from build123d import *

# Parameters (mm, degrees)
CROQUIS1_R              = 10.668
SALIENTE_EXTRUIR1_DEPTH = 5
CROQUIS7_W              = 2
CROQUIS7_H              = 8
CORTAR_EXTRUIR5_DEPTH   = 44.28049503
SALIENTE_EXTRUIR3_DEPTH = 10
CORTAR_EXTRUIR6_REACH   = 53.457
CROQUIS9_R              = 2.25
SALIENTE_EXTRUIR4_DEPTH = 10
CROQUIS11_W             = 29.05
CROQUIS11_H             = 10
SALIENTE_EXTRUIR5_DEPTH = 5
CORTAR_EXTRUIR7_REACH   = 52.054
SALIENTE_EXTRUIR6_DEPTH = 8.51
CORTAR_EXTRUIR8_REACH   = 58.395
SALIENTE_EXTRUIR7_DEPTH = 5


with BuildPart() as part:
    # Croquis1 → Saliente-Extruir1 (new, symmetric)
    with BuildSketch(Plane(origin=(0, 0, 0), x_dir=(1, 0, 0), z_dir=(0, 1, 0))):
        with BuildLine():
            Line((14.525, 0), (-14.525, 0))
            Line((-14.525, 0), (-14.525, -10))
            Line((-14.525, -10), (-5, -10))
            Line((-5, -10), (-5, -11.362711963))
            ThreePointArc((-5, -11.362711963), (0, -39.525), (5, -11.362711963))
            Line((5, -11.362711963), (5, -10))
            Line((5, -10), (14.525, -10))
            Line((14.525, -10), (14.525, 0))
        make_face()
        with Locations(Location((0, -25, 0), (0, 0, 270))):
            Circle(CROQUIS1_R, mode=Mode.SUBTRACT)
    extrude(amount=SALIENTE_EXTRUIR1_DEPTH, both=True)

    # Croquis7 → Cortar-Extruir5 (cut, through all)
    with BuildSketch(Plane(origin=(0, 5, 0), x_dir=(1, 0, 0), z_dir=(0, 1, 0))):
        with Locations((0, -37.5965)):
            Rectangle(CROQUIS7_W, CROQUIS7_H)
    extrude(amount=-CORTAR_EXTRUIR5_DEPTH, mode=Mode.SUBTRACT)

    # Croquis8 → Saliente-Extruir3 (add)
    with BuildSketch(Plane(origin=(0, 5, 0), x_dir=(1, 0, 0), z_dir=(0, 1, 0))):
        with BuildLine():
            Line((-1, -39.490535704), (-1, -45.490535704))
            Line((-1, -45.490535704), (-9, -45.490535704))
            Line((-9, -45.490535704), (-9, -36.400685286))
            ThreePointArc((-9, -36.400685286), (-5.233239332, -38.549495603), (-1, -39.490535704))
        make_face()
        with BuildLine():
            Line((9, -45.490535704), (9, -36.400685286))
            ThreePointArc((9, -36.400685286), (5.233239332, -38.549495603), (1, -39.490535704))
            Line((1, -39.490535704), (1, -45.490535704))
            Line((1, -45.490535704), (9, -45.490535704))
        make_face()
    extrude(amount=-SALIENTE_EXTRUIR3_DEPTH)

    # Cortar-Extruir6: up to this face of the body (flat: up to its plane)
    cortar_extruir6_end = Plane(part.part.faces().sort_by_distance((-9, 0, 40.945610495))[0])
    # Croquis9 → Cortar-Extruir6 (cut, up to the picked face)
    with BuildSketch(Plane(origin=(9, 0, 0), x_dir=(0, 0, -1), z_dir=(1, 0, 0)), mode=Mode.PRIVATE) as cortar_extruir6_sk1:
        with Locations((-40.945610495, 0)):
            Circle(CROQUIS9_R)
    cortar_extruir6_tool1 = split(extrude(cortar_extruir6_sk1.sketch, amount=-CORTAR_EXTRUIR6_REACH, mode=Mode.PRIVATE), bisect_by=cortar_extruir6_end, keep=Keep.BOTH, mode=Mode.PRIVATE)
    add(cortar_extruir6_tool1.solids().sort_by(Axis((9, 0, 40.94561), (-1, 0, 0)))[0], mode=Mode.SUBTRACT)

    # Croquis10 → Saliente-Extruir4 (add)
    with BuildSketch(Plane(origin=(0, 5, 0), x_dir=(1, 0, 0), z_dir=(0, 1, 0))):
        with BuildLine():
            Line((-14.525, -10), (-14.525, -25))
            ThreePointArc((-14.525, -25), (-11.907993639, -16.682830259), (-5, -11.362711963))
            Line((-5, -11.362711963), (-5, -10))
            Line((-5, -10), (-14.525, -10))
        make_face()
        with BuildLine():
            Line((14.525, -10), (5, -10))
            Line((5, -10), (5, -11.362711963))
            ThreePointArc((5, -11.362711963), (11.907993639, -16.682830259), (14.525, -25))
            Line((14.525, -25), (14.525, -10))
        make_face()
    extrude(amount=-SALIENTE_EXTRUIR4_DEPTH)

    # Croquis11 → Saliente-Extruir5 (add)
    with BuildSketch(Plane(origin=(0, 0, 0), x_dir=(-1, 0, 0), z_dir=(0, 0, -1))):
        with Locations((0, 10)):
            Rectangle(CROQUIS11_W, CROQUIS11_H)
    saliente_extruir5 = extrude(amount=-SALIENTE_EXTRUIR5_DEPTH)

    # Croquis13 → Cortar-Extruir7 (cut, up to next)
    with BuildSketch(Plane(origin=(0, 0, 0), x_dir=(-1, 0, 0), z_dir=(0, 0, -1)), mode=Mode.PRIVATE) as cortar_extruir7_sk1:
        with BuildLine():
            Line((1.59, 12.065), (1.59, 15))
            Line((1.59, 15), (3.99, 15))
            Line((3.99, 15), (3.99, 12.065))
            ThreePointArc((3.99, 12.065), (2.79, 10.865), (1.59, 12.065))
        make_face()
    cortar_extruir7_tool1 = extrude(cortar_extruir7_sk1.sketch, amount=-CORTAR_EXTRUIR7_REACH, mode=Mode.PRIVATE) & part.part
    cortar_extruir7 = cortar_extruir7_tool1.solids().sort_by_distance((-2.79, 13.052011, 0))[0]
    add(cortar_extruir7, mode=Mode.SUBTRACT)

    # Simetría1: Saliente-Extruir5, Cortar-Extruir7 across plane
    add(saliente_extruir5.mirror(Plane.ZX))
    add(cortar_extruir7.mirror(Plane.ZX), mode=Mode.SUBTRACT)

    # Croquis14 → Saliente-Extruir6 (add)
    with BuildSketch(Plane(origin=(0, 0, 0), x_dir=(-1, 0, 0), z_dir=(0, 0, -1))):
        Polygon((1.59, -13.71), (-6.6, -13.71), (-6.6, 13.71), (1.59, 13.71), (1.59, 15), (-8.14, 15), (-8.14, -15), (1.59, -15), align=None)
        Polygon((6.6, -13.71), (3.99, -13.71), (3.99, -15), (8.14, -15), (8.14, 15), (3.99, 15), (3.99, 13.71), (6.6, 13.71), align=None)
    extrude(amount=SALIENTE_EXTRUIR6_DEPTH)

    # Croquis15 → Cortar-Extruir8 (cut, up to next)
    with BuildSketch(Plane.XZ.offset(15), mode=Mode.PRIVATE) as cortar_extruir8_sk1:
        with BuildLine():
            Line((4.29, -3.61), (4.29, -8.51))
            Line((4.29, -8.51), (-1.59, -8.51))
            Line((-1.59, -8.51), (-1.59, -0.85))
            Line((-1.59, -0.85), (1.53, -0.85))
            ThreePointArc((1.53, -0.85), (3.481614716, -1.658385284), (4.29, -3.61))
        make_face()
    cortar_extruir8_tool1 = extrude(cortar_extruir8_sk1.sketch, amount=-CORTAR_EXTRUIR8_REACH, mode=Mode.PRIVATE) & part.part
    add(cortar_extruir8_tool1.solids().sort_by_distance((1.262493, -15, -4.801026))[0], mode=Mode.SUBTRACT)

    # Croquis16 → Saliente-Extruir7 (add)
    with BuildSketch(Plane.ZY.offset(14.525)):
        Polygon((5, 15), (15, 5), (5, 5), align=None)
        Polygon((15, -5), (5, -5), (5, -15), align=None)
    saliente_extruir7 = extrude(amount=-SALIENTE_EXTRUIR7_DEPTH)

    # Simetría2: Saliente-Extruir7 across plane
    add(saliente_extruir7.mirror(Plane(origin=(0, 0, 0), x_dir=(0, 0, 1), z_dir=(1, 0, 0))))


solid = part.part
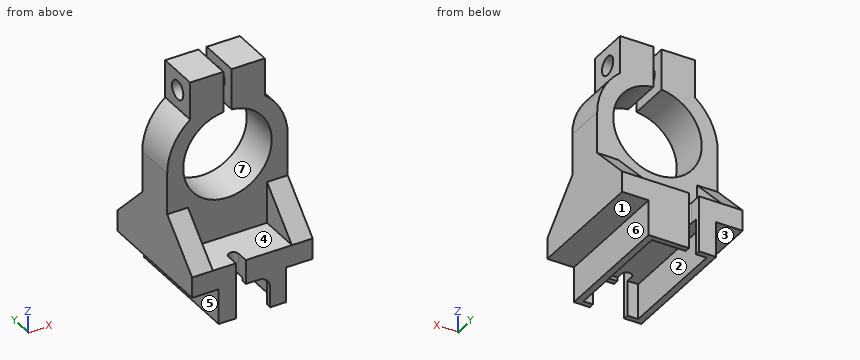
Verification items for the finished model (mm, model axes). Face numbers are marked on the shaded views. A direction names the side the tool comes from. Coordinates: 2 decimals unless noted, no trailing zeros. Loops run counter-clockwise (first coordinate to the right, second up) from the corner with the lowest first, then second, coordinate; pieces in that order, holes last. Notation, with made-up numbers: (-33.75, 51) -> (-21.75, 51) arc R20 ccw to (-21.75, 87) -> close; hole circle Ø5 at (78, -38). An arc over 180 degrees is marked (long way). Answer as a JSON object with one key per item and string values. Group by question number.
Item 1: Tool access check on the marked faces 1, 2, 3 and 4. Record the directions out of +Z, -Z, +X, -X, +Y, -Y that give a thin tool (end or side, any length) a straight path to the whole face; none if there is none.
Item 2: Sectioned sample at B-B on x = -2.79. Record the boundary of the cut face in (y, z) (3 decimals).
Item 3: Sectioned sample at A-A on y = 0. Record the boundary of the cut face in (x, z) (3 decimals).
Item 4: Sectioned sample at C-C on z = 34. Record the boundary of the cut face in (x, y).
Item 5: Depth check by flat-ended pin: pin 1 (5 mm diameter, centred on x = -3, y = -11.5, fed in from +Z); pin 2 (12 mm diameter, centred on x = -6, z = 33.5, fed in from +Y); pin 3 (6 mm diameter, centred on y = 0, z = 40.95, fed in from -X). Enter the tip coordinate at first touch or a pass-through.
Item 6: Sectioned sample at D-D on y = -9.5. Record the boundary of the cut face in (x, z) (3 decimals).
Item 7: Mould release check, pull along X, two halves, no side actions. Record for the marked faces 5, 6 and 7: +X half, -X half, draft (parallel to the pull), parting line (faces both ways), or undercut.
Item 8: Scan lines: probe 1 along X at (y, z) = (-4.75, -5); probe 2 along X at (y, z) = (6.25, 12.5) (3 decimals); probe 3 along Z at (x, y) = (-8.25, 13). Record each from-to range of solid material in increasing order.
Evaluation:
{
 "1": {"face 1": "-Z, +X, +Y, -Y", "face 2": "-Z", "face 3": "-Z, -X, +Y, -Y", "face 4": "+Z, -Y"},
 "2": {"outline": "(-10.865, 0) -> (10.865, 0) -> (10.865, 5) -> (5, 5) -> (5, 14.703) -> (-5, 14.703) -> (-5, 5) -> (-10.865, 5) -> close; (-5, 35.297) -> (5, 35.297) -> (5, 45.491) -> (-5, 45.491) -> close; hole circle Ø4.5 at (0, 40.946)"},
 "3": {"outline": "(-14.525, 0) -> (-8.14, 0) -> (-8.14, -8.51) -> (-6.6, -8.51) -> (-6.6, 0) -> (6.6, 0) -> (6.6, -8.51) -> (8.14, -8.51) -> (8.14, 0) -> (14.525, 0) -> (14.525, 25) arc R14.525 ccw to (9, 36.401) -> (9, 38.696) -> (1, 38.696) -> (1, 35.621) arc R10.668 cw (long way) to (-1, 35.621) -> (-1, 38.696) -> (-9, 38.696) -> (-9, 36.401) arc R14.525 ccw to (-14.525, 25) -> close; (-9, 43.196) -> (-1, 43.196) -> (-1, 45.491) -> (-9, 45.491) -> close; (1, 43.196) -> (9, 43.196) -> (9, 45.491) -> (1, 45.491) -> close"},
 "4": {"outline": "(-11.4, -5) -> (-5.73, -5) -> (-5.73, 5) -> (-11.4, 5) -> close; (5.73, -5) -> (11.4, -5) -> (11.4, 5) -> (5.73, 5) -> close"},
 "5": {"pin 1": "stops at z = 5", "pin 2": "stops at y = 5", "pin 3": "stops at x = -9"},
 "6": {"outline": "(-14.525, 0) -> (-8.14, 0) -> (-8.14, -8.51) -> (-6.6, -8.51) -> (-6.6, 0) -> (6.6, 0) -> (6.6, -8.51) -> (8.14, -8.51) -> (8.14, 0) -> (14.525, 0) -> (14.525, 10.5) -> (9.525, 10.5) -> (9.525, 5) -> (-9.525, 5) -> (-9.525, 10.5) -> (-14.525, 10.5) -> close"},
 "7": {"face 5": "-X half", "face 6": "+X half", "face 7": "undercut"},
 "8": {"probe 1": "x = -8.14 to -6.6, 6.6 to 8.14", "probe 2": "x = -14.525 to -9.525, 9.525 to 14.525", "probe 3": "z = 0 to 5"}
}
